Work out the finished part from the listing and answer in its coordinate system (mm). Give positions to 0.01 mm unless a question says otherwise; leave off trailing zeros. Loops run counter-clockwise (first coordinate to the right, second up) from the corner with the lowest first, then second, coordinate; pieces in that order, holes last. Notation, with made-up numbers: M 68.5,70.5 L 77.5,70.5 A22 ccw 77.5,101.5 Z; hole C -21,7.25 d11. An arc over 180 degrees is marked long. Answer as a JSON object with one key per item and string values. Group by question number.
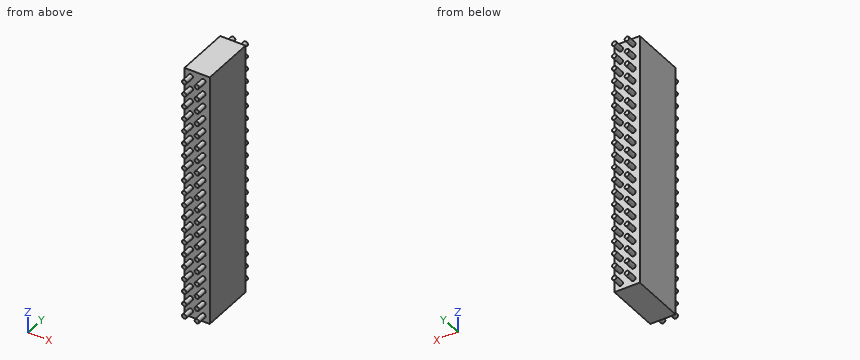
```python
from build123d import *

# Parameters (mm, degrees)
SKIZZE1_W                            = 5.08
SKIZZE1_H                            = 50.8
AUFSATZ_LINEAR_AUSTRAGEN1_DEPTH      = 11
SKIZZE2_R                            = 0.45
AUFSATZ_LINEAR_AUSTRAGEN2_DEPTH      = 2
AUFSATZ_LINEAR_AUSTRAGEN2_DEPTH_BACK = 13


with BuildPart() as part:
    # Skizze1 → Aufsatz-Linear austragen1 (new body)
    with BuildSketch(Plane(origin=(0, 0, 0), x_dir=(1, 0, 0), z_dir=(0, 1, 0))):
        with Locations((2.54, 25.4)):
            Rectangle(SKIZZE1_W, SKIZZE1_H)
    extrude(amount=AUFSATZ_LINEAR_AUSTRAGEN1_DEPTH)

    # Skizze2 → Aufsatz-Linear austragen2 (add, two sides)
    with BuildSketch(Plane(origin=(0, 11, 0), x_dir=(1, 0, 0), z_dir=(0, 1, 0))) as aufsatz_linear_austragen2_sk:
        with Locations((1.27, 1.27)):
            Circle(SKIZZE2_R)
        with Locations((3.81, 1.27)):
            Circle(SKIZZE2_R)
        with Locations((3.81, 3.81)):
            Circle(SKIZZE2_R)
        with Locations((3.81, 6.35)):
            Circle(SKIZZE2_R)
        with Locations((3.81, 8.89)):
            Circle(SKIZZE2_R)
        with Locations((3.81, 11.43)):
            Circle(SKIZZE2_R)
        with Locations((3.81, 13.97)):
            Circle(SKIZZE2_R)
        with Locations((3.81, 16.51)):
            Circle(SKIZZE2_R)
        with Locations((3.81, 19.05)):
            Circle(SKIZZE2_R)
        with Locations((3.81, 21.59)):
            Circle(SKIZZE2_R)
        with Locations((3.81, 24.13)):
            Circle(SKIZZE2_R)
        with Locations((1.27, 3.81)):
            Circle(SKIZZE2_R)
        with Locations((1.27, 6.35)):
            Circle(SKIZZE2_R)
        with Locations((1.27, 8.89)):
            Circle(SKIZZE2_R)
        with Locations((1.27, 11.43)):
            Circle(SKIZZE2_R)
        with Locations((1.27, 13.97)):
            Circle(SKIZZE2_R)
        with Locations((1.27, 16.51)):
            Circle(SKIZZE2_R)
        with Locations((1.27, 19.05)):
            Circle(SKIZZE2_R)
        with Locations((1.27, 21.59)):
            Circle(SKIZZE2_R)
        with Locations((1.27, 24.13)):
            Circle(SKIZZE2_R)
        with Locations((1.27, 26.67)):
            Circle(SKIZZE2_R)
        with Locations((3.81, 26.67)):
            Circle(SKIZZE2_R)
        with Locations((1.27, 29.21)):
            Circle(SKIZZE2_R)
        with Locations((3.81, 29.21)):
            Circle(SKIZZE2_R)
        with Locations((1.27, 31.75)):
            Circle(SKIZZE2_R)
        with Locations((3.81, 31.75)):
            Circle(SKIZZE2_R)
        with Locations((1.27, 34.29)):
            Circle(SKIZZE2_R)
        with Locations((3.81, 34.29)):
            Circle(SKIZZE2_R)
        with Locations((1.27, 36.83)):
            Circle(SKIZZE2_R)
        with Locations((3.81, 36.83)):
            Circle(SKIZZE2_R)
        with Locations((1.27, 39.37)):
            Circle(SKIZZE2_R)
        with Locations((3.81, 39.37)):
            Circle(SKIZZE2_R)
        with Locations((1.27, 41.91)):
            Circle(SKIZZE2_R)
        with Locations((3.81, 41.91)):
            Circle(SKIZZE2_R)
        with Locations((1.27, 44.45)):
            Circle(SKIZZE2_R)
        with Locations((3.81, 44.45)):
            Circle(SKIZZE2_R)
        with Locations((1.27, 46.99)):
            Circle(SKIZZE2_R)
        with Locations((3.81, 46.99)):
            Circle(SKIZZE2_R)
        with Locations((1.27, 49.53)):
            Circle(SKIZZE2_R)
        with Locations((3.81, 49.53)):
            Circle(SKIZZE2_R)
    extrude(amount=AUFSATZ_LINEAR_AUSTRAGEN2_DEPTH)
    extrude(aufsatz_linear_austragen2_sk.sketch, amount=-AUFSATZ_LINEAR_AUSTRAGEN2_DEPTH_BACK)


solid = part.part
```
Item 1: Find the intervals of material crossed by probe 1 along Y at (x, z) = (1.4, -46.5); probe 2 along X at (y, z) = (-0.25, -9), in increasing order. Write a range as [from, to].
Item 2: A cutting plane is placed at B-B (y = 12). Give the number of separate pieces and of enclosed holes in the cut face, and give its area (3 significant figures).
Item 3: A cutting plane is placed at A-A (z = -46.99). Determine the outline of the cut face in (x, y).
Item 4: A cutting plane is placed at C-C (x = 2.45). Determine the outline of the cut face in (y, z), and give its area (3 significant figures).
Item 5: Given pin 1 Ø3 at (x, z) = (2.5, -7.5) entering from +Y, flat-ended and moving along its own axis, determine where the tip first touches the part or whether it passes through.
The answers:
{
 "1": {"probe 1": "y = [0, 11]", "probe 2": "x = [0.83, 1.71], [3.37, 4.25]"},
 "2": {"separate pieces": "40", "enclosed holes": "0", "area": "25.4 mm^2"},
 "3": {"outline": "M 0,0 L 0.82,0 L 0.82,-2 L 1.72,-2 L 1.72,0 L 3.36,0 L 3.36,-2 L 4.26,-2 L 4.26,0 L 5.08,0 L 5.08,11 L 4.26,11 L 4.26,13 L 3.36,13 L 3.36,11 L 1.72,11 L 1.72,13 L 0.82,13 L 0.82,11 L 0,11 Z"},
 "4": {"outline": "M 0,-50.8 L 11,-50.8 L 11,0 L 0,0 Z", "area": "559 mm^2"},
 "5": {"pin 1": "stops at y = 13"}
}
